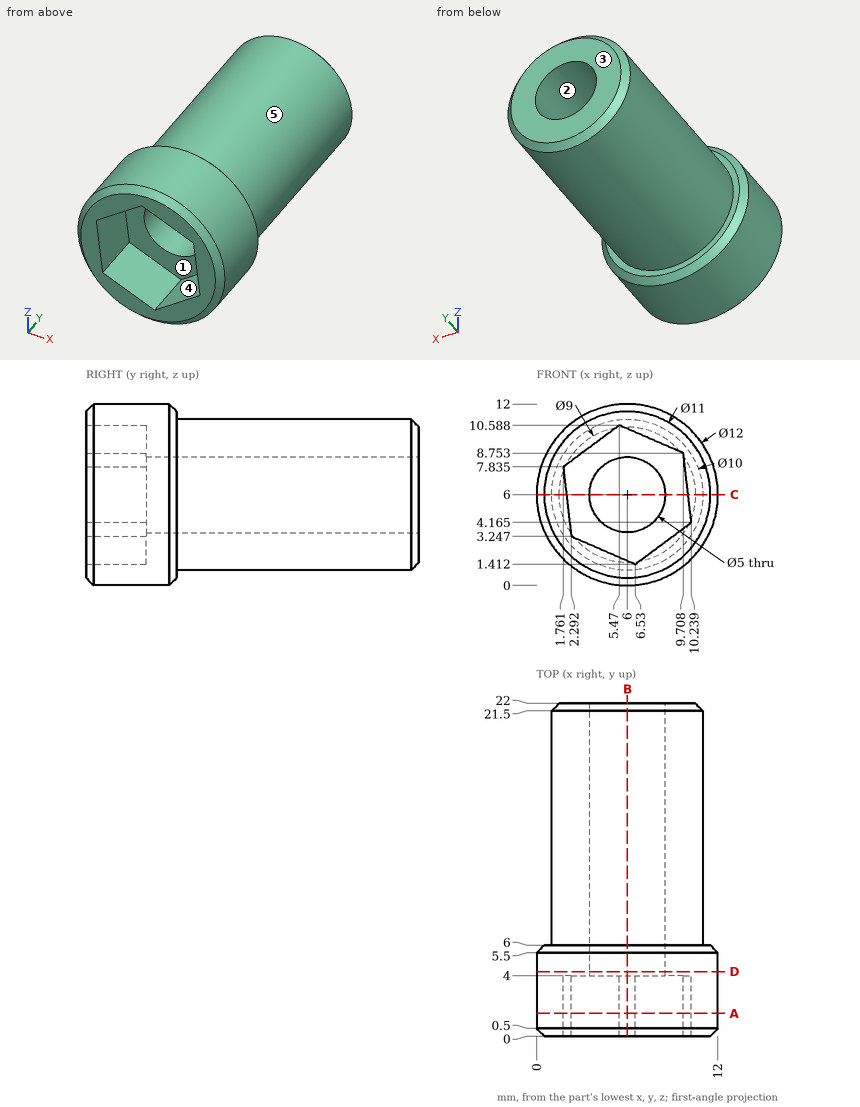
Print and shaded views of the part. All mm, measured from the part's lowest x, y and z. A direction names the side the tool comes from. Give positions to 0.01 mm unless a question says otherwise; leave off trailing zeros. Loops run counter-clockwise (first coordinate to the right, second up) from the corner with the lowest first, then second, coordinate; pieces in that order, holes last. Notation, with made-up numbers: (80.5, 74) -> (104.5, 74) arc R11 cw to (104.5, 82) -> close; hole circle Ø6 at (9, 54.5). An arc over 180 degrees is marked (long way). Use CSV: the item, a comma, the result in double quotes. Start each with the question number.
1) Flat gauge pins, fed straight in: pin 1 Ø5 at (y, z) = (5, 1.5) entering from +X; pin 2 Ø6 at (x, z) = (6, 6) entering from -Y; pin 3 Ø1.5 at (x, z) = (10, 1.5) entering from +Y. Where does each tip first touch, or does it go through?
2) Wall check: line 1 (Z direction, x = 6, y = 14.75); line 2 (Y direction, x = 3.5, z = 5); line 3 (X direction, y = 4.25, z = 4.25) (1 decimal). Give the ranges that are in metal, low to high.
3) Tool access for the marked faces 1 and 2: list every direction of +Z, -Z, +X, -X, +Y, -Y with a clear straight run to the whole face (end or side of a thin tool).
4) Slice it at C-C on z = 6. Give the cut face in (x, y), plus the area to 3 significant figures.
5) Slice it at B-B on x = 6. Give the cut face in (y, z).
6) Slice it at D-D on y = 4.25. Give the cut face in (x, z).
7) Mould opens along X. For the marked faces 3, 4 and 5 say: released by +X, released by -X, zero draft, split by the parting line, or undercut.
8) Slice it at A-A on y = 1.5. Give the cut face in (x, z) (1 decimal).
Computed values:
1,pin 1,"stops at x = 11.66"
1,pin 2,"stops at y = 4"
1,pin 3,"stops at y = 6"
2,line 1,"z = 1 to 3.5, 8.5 to 11"
2,line 2,"y = 4 to 22"
2,line 3,"x = 0.3 to 4.2, 7.8 to 11.7"
3,face 1,"-Y"
3,face 2,"+Y, -Y"
4,outline,"(0, 0.5) -> (0.5, 0) -> (1.97, 0) -> (1.97, 4) -> (3.5, 4) -> (3.5, 22) -> (1.5, 22) -> (1, 21.5) -> (1, 6) -> (0.5, 6) -> (0, 5.5) -> close; (8.5, 4) -> (10.03, 4) -> (10.03, 0) -> (11.5, 0) -> (12, 0.5) -> (12, 5.5) -> (11.5, 6) -> (11, 6) -> (11, 21.5) -> (10.5, 22) -> (8.5, 22) -> close"
4,area,"109 mm^2"
5,outline,"(0, 0.5) -> (0.5, 0) -> (5.5, 0) -> (6, 0.5) -> (6, 1) -> (21.5, 1) -> (22, 1.5) -> (22, 3.5) -> (4, 3.5) -> (4, 1.64) -> (0, 1.64) -> close; (0, 10.36) -> (4, 10.36) -> (4, 8.5) -> (22, 8.5) -> (22, 10.5) -> (21.5, 11) -> (6, 11) -> (6, 11.5) -> (5.5, 12) -> (0.5, 12) -> (0, 11.5) -> close"
6,outline,"circle Ø12 at (6, 6); hole circle Ø5 at (6, 6)"
7,face 3,"zero draft"
7,face 4,"undercut"
7,face 5,"split by the parting line"
8,outline,"circle Ø12 at (6, 6); hole (1.8, 7.8) -> (2.3, 3.2) -> (6.5, 1.4) -> (10.2, 4.2) -> (9.7, 8.8) -> (5.5, 10.6) -> close"
